from build123d import *

# Parameters (mm, degrees)
SKETCH1_W            = 150
SKETCH1_H            = 150
BOSS_EXTRUDE1_DEPTH  = 7.5
SKETCH2_W            = 150
SKETCH2_H            = 150
SKETCH2_W_2          = 135
SKETCH2_H_2          = 135
BOSS_EXTRUDE2_DEPTH  = 92.5
SKETCH3_W            = 20
SKETCH3_H            = 10
BOSS_EXTRUDE3_DEPTH  = 65
SKETCH4_R            = 5.8075
BOSS_EXTRUDE4_DEPTH  = 15
SKETCH5_W            = 9.35632758
SKETCH5_H            = 19.933045712
BOSS_EXTRUDE5_DEPTH  = 65
SKETCH7_W            = 7.5
SKETCH7_H            = 5
SKETCH7_W_2          = 10
BOSS_EXTRUDE7_DEPTH  = 65
SKETCH8_R            = 2.5
BOSS_EXTRUDE8_DEPTH  = 17.5
SKETCH10_W           = 17.5
SKETCH10_H           = 5
BOSS_EXTRUDE10_DEPTH = 65
SKETCH12_R           = 3
BOSS_EXTRUDE11_DEPTH = 20
SKETCH6_R            = 3
CUT_EXTRUDE1_DEPTH   = 10
SKETCH13_W           = 16
SKETCH13_H           = 12
BOSS_EXTRUDE12_DEPTH = 12.5
SKETCH14_W           = 35
SKETCH14_H           = 41
BOSS_EXTRUDE13_DEPTH = 31
SKETCH15_R           = 5
CUT_EXTRUDE2_DEPTH   = 10
SKETCH16_W           = 150
SKETCH16_H           = 5
BOSS_EXTRUDE14_DEPTH = 5
SKETCH17_W           = 12.5
SKETCH17_H           = 5
SKETCH17_W_2         = 50
BOSS_EXTRUDE15_DEPTH = 5
SKETCH18_W           = 150
SKETCH18_H           = 5
BOSS_EXTRUDE16_DEPTH = 5
SKETCH19_W           = 150
SKETCH19_H           = 5
BOSS_EXTRUDE17_DEPTH = 5
SKETCH20_R           = 2.5
CUT_EXTRUDE3_DEPTH   = 10
SKETCH21_R           = 2.5
CUT_EXTRUDE4_DEPTH   = 10
SKETCH22_R           = 1.5
CUT_EXTRUDE5_DEPTH   = 5
SKETCH23_R           = 1
SKETCH23_R_2         = 0.6
CUT_EXTRUDE6_DEPTH   = 4
SKETCH24_R           = 0.75
SKETCH24_R_2         = 0.5
CUT_EXTRUDE7_DEPTH   = 4


with BuildPart() as part:
    # Sketch1 → Boss-Extrude1 (new body)
    with BuildSketch(Plane(origin=(0, 0, 0), x_dir=(1, 0, 0), z_dir=(0, 1, 0))):
        Rectangle(SKETCH1_W, SKETCH1_H)
    extrude(amount=BOSS_EXTRUDE1_DEPTH)

    # Sketch2 → Boss-Extrude2 (add)
    with BuildSketch(Plane(origin=(0, 7.5, 0), x_dir=(1, 0, 0), z_dir=(0, 1, 0))):
        Rectangle(SKETCH2_W, SKETCH2_H)
        Rectangle(SKETCH2_W_2, SKETCH2_H_2, mode=Mode.SUBTRACT)
    extrude(amount=BOSS_EXTRUDE2_DEPTH)

    # Sketch3 → Boss-Extrude3 (add)
    with BuildSketch(Plane(origin=(0, 7.5, 0), x_dir=(1, 0, 0), z_dir=(0, 1, 0))):
        with Locations((0, 57.724473197)):
            Rectangle(SKETCH3_W, SKETCH3_H)
    extrude(amount=BOSS_EXTRUDE3_DEPTH)

    # Sketch4 → Boss-Extrude4 (add)
    with BuildSketch(Plane.XY.offset(-52.724473197)):
        with Locations((0, 57.5)):
            Circle(SKETCH4_R)
    extrude(amount=BOSS_EXTRUDE4_DEPTH)

    # Sketch5 → Boss-Extrude5 (add)
    with BuildSketch(Plane(origin=(0, 7.5, 0), x_dir=(1, 0, 0), z_dir=(0, 1, 0))):
        with Locations((-43.5, 27.5)):
            Rectangle(SKETCH5_W, SKETCH5_H)
    extrude(amount=BOSS_EXTRUDE5_DEPTH)

    # Sketch7 → Boss-Extrude7 (add)
    with BuildSketch(Plane(origin=(0, 7.5, 0), x_dir=(1, 0, 0), z_dir=(0, 1, 0))):
        with Locations((-27.25, -2.5)):
            Rectangle(SKETCH7_W, SKETCH7_H)
        with Locations((-18.5, -2.5)):
            Rectangle(SKETCH7_W_2, SKETCH7_H)
    extrude(amount=BOSS_EXTRUDE7_DEPTH)

    # Sketch8 → Boss-Extrude8 (add)
    with BuildSketch(Plane(origin=(0, 0, 0), x_dir=(-1, 0, 0), z_dir=(0, 0, -1))):
        with Locations((20, 57.5)):
            Circle(SKETCH8_R)
    extrude(amount=BOSS_EXTRUDE8_DEPTH)

    # Sketch10 → Boss-Extrude10 (add)
    with BuildSketch(Plane(origin=(0, 7.5, 0), x_dir=(1, 0, 0), z_dir=(0, 1, 0))):
        with Locations((-22.25, 2.5)):
            Rectangle(SKETCH10_W, SKETCH10_H)
    extrude(amount=BOSS_EXTRUDE10_DEPTH)

    # Sketch12 → Boss-Extrude11 (add)
    with BuildSketch(Plane(origin=(-13.5, 0, 0), x_dir=(0, 0, -1), z_dir=(1, 0, 0))):
        with Locations((0, 57.5)):
            Circle(SKETCH12_R)
    extrude(amount=BOSS_EXTRUDE11_DEPTH)

    # Sketch6 → Cut-Extrude1 (cut)
    with BuildSketch(Plane(origin=(-38.82183621, 0, 0), x_dir=(0, 0, -1), z_dir=(1, 0, 0))):
        with Locations((27.466522856, 57.5)):
            Circle(SKETCH6_R)
    extrude(amount=-CUT_EXTRUDE1_DEPTH, mode=Mode.SUBTRACT)

    # Sketch13 → Boss-Extrude12 (add)
    with BuildSketch(Plane(origin=(0, 7.5, 0), x_dir=(1, 0, 0), z_dir=(0, 1, 0))):
        with Locations((26.2, 27.5)):
            Rectangle(SKETCH13_W, SKETCH13_H)
    extrude(amount=BOSS_EXTRUDE12_DEPTH)

    # Sketch14 → Boss-Extrude13 (add)
    with BuildSketch(Plane(origin=(0, 7.5, 0), x_dir=(1, 0, 0), z_dir=(0, 1, 0))):
        with Locations((47.5, 13)):
            Rectangle(SKETCH14_W, SKETCH14_H)
    extrude(amount=BOSS_EXTRUDE13_DEPTH)

    # Sketch15 → Cut-Extrude2 (cut)
    with BuildSketch(Plane(origin=(75, 0, 0), x_dir=(0, 0, -1), z_dir=(1, 0, 0))):
        with Locations((27.466523, 57.5)):
            Circle(SKETCH15_R)
    extrude(amount=-CUT_EXTRUDE2_DEPTH, mode=Mode.SUBTRACT)

    # Sketch16 → Boss-Extrude14 (add)
    with BuildSketch(Plane(origin=(0, 0, 67.5), x_dir=(-1, 0, 0), z_dir=(0, 0, -1))):
        with Locations((0, 91.5)):
            Rectangle(SKETCH16_W, SKETCH16_H)
    extrude(amount=BOSS_EXTRUDE14_DEPTH)

    # Sketch17 → Boss-Extrude15 (add)
    with BuildSketch(Plane.XY.offset(-67.5)):
        with Locations((-61.25, 91.5)):
            Rectangle(SKETCH17_W, SKETCH17_H)
        with Locations((0, 91.5)):
            Rectangle(SKETCH17_W_2, SKETCH17_H)
        with Locations((61.25, 91.5)):
            Rectangle(SKETCH17_W, SKETCH17_H)
    extrude(amount=BOSS_EXTRUDE15_DEPTH)

    # Sketch18 → Boss-Extrude16 (add)
    with BuildSketch(Plane.ZY.offset(-67.5)):
        with Locations((0, 91.5)):
            Rectangle(SKETCH18_W, SKETCH18_H)
    extrude(amount=BOSS_EXTRUDE16_DEPTH)

    # Sketch19 → Boss-Extrude17 (add)
    with BuildSketch(Plane(origin=(-67.5, 0, 0), x_dir=(0, 0, -1), z_dir=(1, 0, 0))):
        with Locations((0, 91.5)):
            Rectangle(SKETCH19_W, SKETCH19_H)
    extrude(amount=BOSS_EXTRUDE17_DEPTH)

    # Sketch20 → Cut-Extrude3 (cut)
    with BuildSketch(Plane(origin=(0, 0, -75), x_dir=(-1, 0, 0), z_dir=(0, 0, -1))):
        with Locations((-50, 85)):
            Circle(SKETCH20_R)
        with Locations((-40, 85)):
            Circle(SKETCH20_R)
        with Locations((-30, 85)):
            Circle(SKETCH20_R)
        with Locations((30, 85)):
            Circle(SKETCH20_R)
        with Locations((40, 85)):
            Circle(SKETCH20_R)
        with Locations((50, 85)):
            Circle(SKETCH20_R)
    extrude(amount=-CUT_EXTRUDE3_DEPTH, mode=Mode.SUBTRACT)

    # Sketch21 → Cut-Extrude4 (cut)
    with BuildSketch(Plane.XZ):
        with Locations((-60, 60)):
            Circle(SKETCH21_R)
        with Locations((60, 60)):
            Circle(SKETCH21_R)
        with Locations((-60, -60)):
            Circle(SKETCH21_R)
        with Locations((60, -60)):
            Circle(SKETCH21_R)
    extrude(amount=-CUT_EXTRUDE4_DEPTH, mode=Mode.SUBTRACT)

    # Sketch22 → Cut-Extrude5 (cut)
    with BuildSketch(Plane.XY.offset(75)):
        with Locations((-14.5, 94.75)):
            Circle(SKETCH22_R)
        with Locations((14.5, 94.75)):
            Circle(SKETCH22_R)
    extrude(amount=-CUT_EXTRUDE5_DEPTH, mode=Mode.SUBTRACT)

    # Sketch23 → Cut-Extrude6 (cut)
    with BuildSketch(Plane(origin=(0, 38.5, 0), x_dir=(1, 0, 0), z_dir=(0, 1, 0))):
        with Locations((32.5, 8.61)):
            Circle(SKETCH23_R)
        with Locations((32.5, 27.61)):
            Circle(SKETCH23_R)
        with Locations((63, 31.61)):
            Circle(SKETCH23_R_2)
        with Locations((57, 31.61)):
            Circle(SKETCH23_R_2)
        with Locations((57, 7.31)):
            Circle(SKETCH23_R_2)
        with Locations((63, 7.31)):
            Circle(SKETCH23_R_2)
        with Locations((57, 28.908369489)):
            Circle(SKETCH23_R_2)
        with Locations((63, 28.91)):
            Circle(SKETCH23_R_2)
        with Locations((63, 4.61)):
            Circle(SKETCH23_R_2)
        with Locations((57, 4.61)):
            Circle(SKETCH23_R_2)
    extrude(amount=-CUT_EXTRUDE6_DEPTH, mode=Mode.SUBTRACT)

    # Sketch24 → Cut-Extrude7 (cut)
    with BuildSketch(Plane(origin=(0, 20, 0), x_dir=(1, 0, 0), z_dir=(0, 1, 0))):
        with Locations((23.7, 24.466522856)):
            Circle(SKETCH24_R)
        with Locations((23.7, 30.5)):
            Circle(SKETCH24_R)
        with Locations((19.7, 31.716522856)):
            Circle(SKETCH24_R_2)
        with Locations((19.7, 23.2)):
            Circle(SKETCH24_R_2)
    extrude(amount=-CUT_EXTRUDE7_DEPTH, mode=Mode.SUBTRACT)


solid = part.part
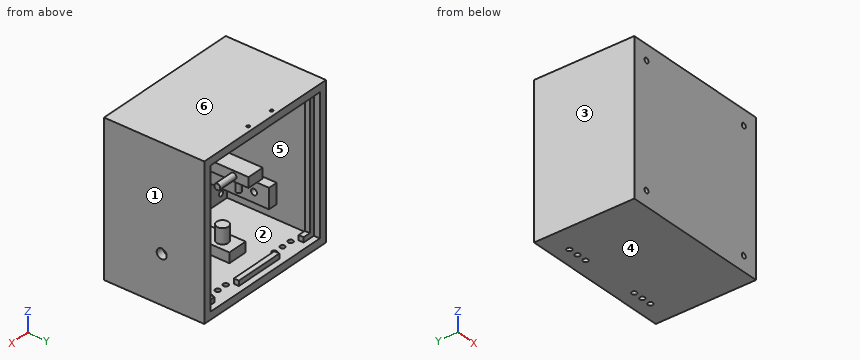
Part model, mm, in its own coordinate system. Face numbers are marked on the shaded views. A direction names the side the tool comes from. Give positions to 0.01 mm unless a question says otherwise; leave off trailing zeros. Loops run counter-clockwise (first coordinate to the right, second up) from the corner with the lowest first, then second, coordinate; pieces in that order, holes last.
(1) Band-saw the part on C-C (x = 0). Write the cut outline in (y, z), and give its area (4 significant figures).
Return value:
outline: (0, -75) - (100, -75) - (100, -67.5) - (94, -67.5) - (94, -62.5) - (89, -62.5) - (89, -67.5) - (7.5, -67.5) - (7.5, -62.72) - (72.5, -62.72) - (72.5, -52.72) - (63.31, -52.72) - (63.31, -37.72) - (51.69, -37.72) - (51.69, -52.72) - (7.5, -52.72) - (7.5, 67.5) - (89, 67.5) - (89, 62.5) - (94, 62.5) - (94, 67.5) - (100, 67.5) - (100, 75) - (0, 75) - close; circle Ø6 at (57.5, 0)
area: 3,415 mm2
(2) Pin check, flat tips, straight feed: pin 1 (1.1 mm diameter, centred on x = 19.5, z = -31.5, fed in from +Y); pin 2 (1 mm diameter, centred on x = 63, z = -31.5, fed in from +Y). Stop position of each tip, or through.
Return value:
pin 1: stops at y = 20
pin 2: stops at y = 94
(3) Band-saw the part on A-A (z = -14). Write the cut outline in (x, y), and give its area (3 significant figures).
Return value:
outline: (-75, 0) - (75, 0) - (75, 100) - (67.5, 100) - (67.5, 94) - (62.5, 94) - (62.5, 89) - (67.5, 89) - (67.5, 7.5) - (65, 7.5) - (65, 38.5) - (30, 38.5) - (30, 7.5) - (-67.5, 7.5) - (-67.5, 89) - (-62.5, 89) - (-62.5, 94) - (-67.5, 94) - (-67.5, 100) - (-75, 100) - close; circle Ø5 at (-20, 57.5)
area: 3,670 mm2
(4) Drill centre lines: line 1 along Z through (x, y) = (8.5, 63); line 2 along Z through (x, y) = (60, 1.75); line 3 along X through (y, z) = (19, -53.5). Where is each one in solid material? Low to high.
Return value:
line 1: z = -75 to -67.5, -62.72 to -52.72, 67.5 to 75
line 2: z = -75 to -62.5, -57.5 to 57.5, 62.5 to 75
line 3: x = -75 to -67.5, -10 to 10, 67.5 to 75
(5) Band-saw the part on D-D (x = 60.5). Write the cut outline in (y, z), and give its area (3 significant figures).
Return value:
outline: (0, -75) - (100, -75) - (100, -67.5) - (94, -67.5) - (94, -62.5) - (89, -62.5) - (89, -67.5) - (7.5, -67.5) - (7.5, -62.45) - (0, -62.45) - close; (0, -57.55) - (7.5, -57.55) - (7.5, -33.5) - (38.5, -33.5) - (38.5, 7.5) - (7.5, 7.5) - (7.5, 57.55) - (0, 57.55) - close; (0, 62.45) - (7.5, 62.45) - (7.5, 67.5) - (89, 67.5) - (89, 62.5) - (94, 62.5) - (94, 67.5) - (100, 67.5) - (100, 75) - (0, 75) - close
area: 3,760 mm2
(6) 3-axis set-ups, long thin cutter, end or side, ignore diameter. For the marked faces 5 and 6: which of +Z, -Z, +X, -X, +Y, -Y reach the whole face in a straight line?
Return value:
face 5: none
face 6: +Z, +X, -X, +Y, -Y
(7) Pull direction X, two halves, no side cores. Call the marked faces 1, 2, 3 and 4: pulls with the +X half, pulls with the -X half, needs draft (parallel to the pull), parting line crosses it, or undercut.
Return value:
face 1: pulls with the +X half
face 2: undercut
face 3: pulls with the -X half
face 4: needs draft
(8) Band-saw the part on B-B (y = 27). Write the cut outline in (x, z), and give its area (3 significant figures).
Return value:
outline: (-75, -75) - (75, -75) - (75, 75) - (-75, 75) - close; (-48.18, -37.47) - (-38.82, -37.47) - (-38.82, -17.53) - (-48.18, -17.53) - close; (-31, -5) - (-13.5, -5) - (-13.5, 5) - (-31, 5) - close; (-10, -62.72) - (10, -62.72) - (10, -52.72) - (-10, -52.72) - close; (30, -33.5) - (65, -33.5) - (65, 7.5) - (30, 7.5) - close; hole (-67.5, -67.5) - (67.5, -67.5) - (67.5, 67.5) - (-67.5, 67.5) - close
area: 6,270 mm2
